Could you check a few things on this drawing? It's one solid part, dimensions in mm from its lowest x, y, z. A direction names the side the tool comes from. Give positions to 0.01 mm unless a question says otherwise; leave off trailing zeros. Order: outer loops, then holes, each group sorted by start corner. A loop starts at its lowest first (then second) coordinate and runs counter-clockwise, first axis right, second up.
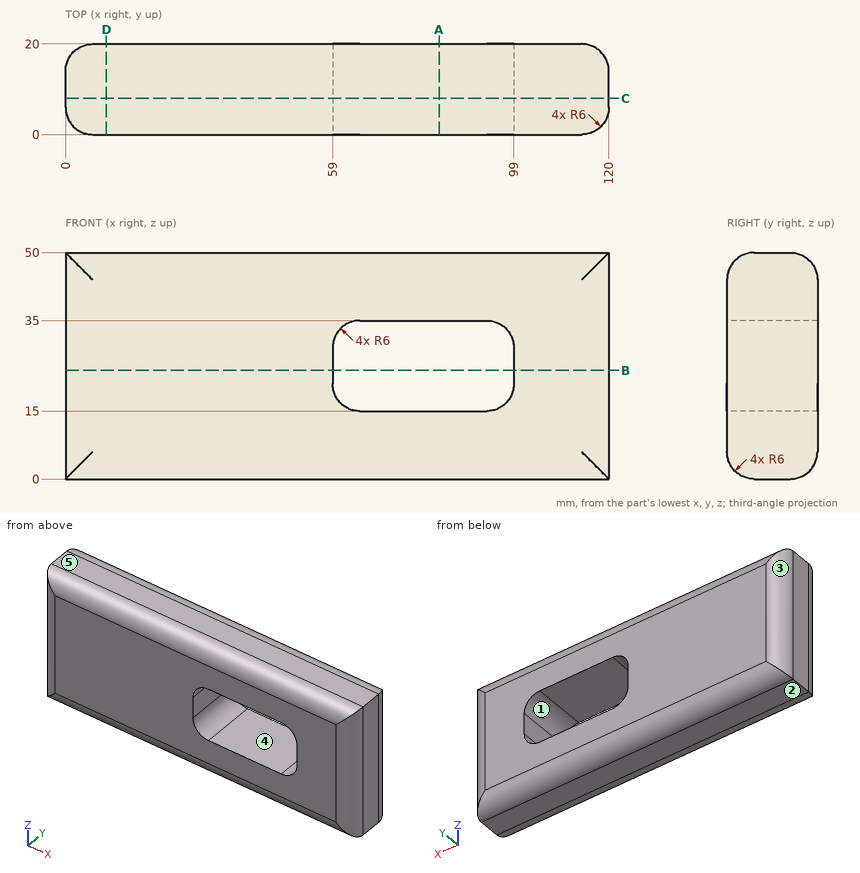
1) Suppose I cut it at B-B (z = 24). Please give me the cut outline in (x, y).
2) Suppose I cut it at D-D (x = 9). Please give me the cut outline in (y, z).
3) Which directions (+Z, -Z, +X, -X, +Y, -Y) give clear straight access to the entire face, cutting with the end or side of a thin tool? Please do the marked faces 4 and 5.
4) I'm going to push flat-ended pins straight in: pin 1 Ø1 at (x, y) = (62, 15.5) entering from +Z; pin 2 Ø1.5 at (y, z) = (4.5, 39.5) entering from -X. Where does each tip first touch, or does it pass through?
5) Suppose I cut it at C-C (y = 8). Please give me the cut outline in (x, z), and give its area (3 significant figures).
6) We'd pull the mould along X, two halves only. Please class the marked faces 1, 2 and 3: +X half, -X half, draft (parallel to the pull), parting line (faces both ways), or undercut.
7) If I drill on line 1 (Z direction, x = 86, y = 11.5); line 2 (X direction, y = 12.5, z = 23); line 3 (Y direction, x = 103, z = 44.5), over which ranges is the centre line in solid material (lowest first)?
8) Suppose I cut it at A-A (x = 82.5). Please give me the cut outline in (y, z), and give its area (3 significant figures).
Results:
1. outline: (0, 6) arc R6 ccw to (6, 0) - (59, 0) - (59, 20) - (6, 20) arc R6 ccw to (0, 14) - close; (99, 0) - (114, 0) arc R6 ccw to (120, 6) - (120, 14) arc R6 ccw to (114, 20) - (99, 20) - close
2. outline: (0, 6) arc R6 ccw to (6, 0) - (14, 0) arc R6 ccw to (20, 6) - (20, 44) arc R6 ccw to (14, 50) - (6, 50) arc R6 ccw to (0, 44) - close
3. face 4: +Y, -Y
3. face 5: +Z, +X, -X, +Y, -Y
4. pin 1: stops at z = 49.92
4. pin 2: stops at x = 0.05
5. outline: (0, 0) - (120, 0) - (120, 50) - (0, 50) - close; hole (59, 21) arc R6 ccw to (65, 15) - (93, 15) arc R6 ccw to (99, 21) - (99, 29) arc R6 ccw to (93, 35) - (65, 35) arc R6 ccw to (59, 29) - close
5. area: 5,230 mm2
6. face 1: undercut
6. face 2: draft
6. face 3: -X half
7. line 1: z = 0 to 15, 35 to 50
7. line 2: x = 0 to 59, 99 to 120
7. line 3: y = 0.02 to 19.98
8. outline: (0, 6) arc R6 ccw to (6, 0) - (14, 0) arc R6 ccw to (20, 6) - (20, 15) - (0, 15) - close; (0, 35) - (20, 35) - (20, 44) arc R6 ccw to (14, 50) - (6, 50) arc R6 ccw to (0, 44) - close
8. area: 569 mm2
